from build123d import *

# Parameters (mm, degrees)
SKETCH1_R           = 3.25
BOSS_EXTRUDE1_DEPTH = 8
FILLET1_R           = 1
SKETCH2_R           = 1.65
CUT_EXTRUDE1_DEPTH  = 5
CUT_EXTRUDE1_DRAFT  = -1.7


with BuildPart() as part:
    # Sketch1 → Boss-Extrude1 (new body)
    with BuildSketch(Plane(origin=(0, 0, 0), x_dir=(1, 0, 0), z_dir=(0, 1, 0))):
        with Locations(Location((0, 0, 0), (0, 0, 270))):
            Circle(SKETCH1_R)
    extrude(amount=BOSS_EXTRUDE1_DEPTH)

    # Fillet1
    fillet1_edges = [part.edges().sort_by_distance(p)[0] for p in [
        (0, 8, -3.25),
    ]]
    fillet(fillet1_edges, radius=FILLET1_R)


with BuildPart() as cut_extrude1_tool:
    # Sketch2 → Cut-Extrude1 (with draft: the straight prism first)
    with BuildSketch(Plane.XZ):
        Circle(SKETCH2_R)
    extrude(amount=-CUT_EXTRUDE1_DEPTH)
    # Cut-Extrude1: the draft: its side faces are tilted about the plane it starts from
    cut_extrude1_sides = [cut_extrude1_tool.faces().sort_by_distance(p)[0] for p in [
        (-1.65, 2.5, 0),
    ]]
    draft(cut_extrude1_sides, Plane.XZ, CUT_EXTRUDE1_DRAFT)


with BuildPart() as part_1:
    add(part.part)

    # Cut-Extrude1: cut by cut_extrude1_tool
    add(cut_extrude1_tool.part, mode=Mode.SUBTRACT)


solid = part_1.part
Source: CAD feature listing. Evaluate the final solid. Frame: model axes, mm. A direction names the side the tool comes from. Round coordinates to 2 decimals unless told otherwise and drop trailing zeros. Loops run counter-clockwise (first coordinate to the right, second up) from the corner with the lowest first, then second, coordinate; pieces in that order, holes last.
Q1. Ray query, line 1 (Y direction, x = 0, z = 0.5); line 2 (X direction, y = 1.75, z = -0.5); line 3 (Z direction, x = 1.25, y = 3.25). Return the intervals inside material, ascending.
Q2. Section C-C, the plane y = 1.5. Return loops of the section in (x, z).
Q3. Section A-A, the plane x = 0. Return loops of the section in (y, z).
Q4. Section B-B, the plane z = 0. Return loops of the section in (x, y), plus the area to 3 significant figures.
Q5. Mould query, pull axis Z, two halves, no side actions, for faces 1 (the face through (-1.978, 3.451, -2.579)), 2 (the face through (1.504, 2.465, 0.474)), 3 (the face through (0, 8, 0)). Classes: pulls with the +Z half, pulls with the -Z half, needs draft (parallel to the pull), parting line crosses it, or undercut.
Q6. First-contact query: P1, Ø1.5, axis at y = 4, z = 1.5, coming from the +X side. Flat tip, straight axial feed; report the tip coordinate or a pass-through.
Q7. Access query for faces 4 (the face through (-1.4, 0, 1.4)), 5 (the face through (0, 5, 0)). Directions: +Z, -Z, +X, -X, +Y, -Y. A direction counts if a zero-diameter tool reaches every point of the face in a straight line with its end or side. Return the directions, or none.
Q8. Section D-D, the plane y = 3.25. Return loops of the section in (x, z), plus the area to 3 significant figures.
Solutions:
1. line 1: y = 5 to 8
1. line 2: x = -3.21 to -1.52, 1.52 to 3.21
1. line 3: z = -3 to -0.92, 0.92 to 3
2. outline: circle Ø6.5 at (0, 0); hole circle Ø3.21 at (0, 0)
3. outline: (0, -3.25) - (7, -3.25) arc R1 ccw to (8, -2.25) - (8, 2.25) arc R1 ccw to (7, 3.25) - (0, 3.25) - (0, 1.65) - (5, 1.5) - (5, -1.5) - (0, -1.65) - close
4. outline: (-3.25, 0) - (-1.65, 0) - (-1.5, 5) - (1.5, 5) - (1.65, 0) - (3.25, 0) - (3.25, 7) arc R1 ccw to (2.25, 8) - (-2.25, 8) arc R1 ccw to (-3.25, 7) - close
4. area: 35.8 mm2
5. face 1: parting line crosses it
5. face 2: undercut
5. face 3: needs draft
6. P1: stops at x = 3.16
7. face 4: +Z, -Z, +X, -X, -Y
7. face 5: -Y
8. outline: circle Ø6.5 at (0, 0); hole circle Ø3.11 at (0, 0)
8. area: 25.6 mm2
